Verification items for the finished model (mm, model axes). Round coordinates to 2 decimals unless told otherwise and drop trailing zeros. Write each question's results on one line, items separated by ' | '.
```python
from build123d import *

# Parameters (mm, degrees)
SKETCH2_R           = 12.7
SKETCH3_R           = 12.7
BOSS_EXTRUDE1_DEPTH = 50
SKETCH4_R           = 12.7
BOSS_EXTRUDE2_DEPTH = 35
SKETCH5_R           = 12.7
CUT_EXTRUDE1_DEPTH  = 634.359519319
SKETCH6_R           = 12.7
BOSS_EXTRUDE3_DEPTH = 40


with BuildPart() as part:
    # Sweep1: sweep along a curve in space
    with BuildLine() as sweep1_path:
        Line((-45.263841099, -132.462271612, 42.727197095), (-9.928000519, -34.667527384, 56.556883965))
        ThreePointArc((-45.263841099, -132.462271612, 42.727197095), (-49.367402807, -154.461340148, 40.074170619), (-46.268448436, -176.708192383, 38.254601427))
        Line((1.796645732, -332.656119714, 28.636985574), (-46.268448436, -176.708192383, 38.254601427))
        ThreePointArc((1.796645732, -332.656119714, 28.636985574), (9.693780672, -349.82422739, 28.096448926), (21.793712602, -364.33648604, 28.718411529))
        Line((159.088704017, -490.606286781, 40.497494579), (21.793712602, -364.33648604, 28.718411529))
        Line((159.088704017, -490.606286781, 40.497494579), (-47.055147145, -424.175155849, 20.376642682))
        ThreePointArc((-47.055147145, -424.175155849, 20.376642682), (-68.707848435, -412.682375082, 18.540437025), (-85.12514007, -394.403432402, 17.735499766))
        Line((-85.12514007, -394.403432402, 17.735499766), (-237.067860888, -150.281613827, 14.887673564))
        ThreePointArc((-237.067860888, -150.281613827, 14.887673564), (-245.860225068, -128.979461941, 14.519507014), (-247.259590984, -105.981912067, 13.905207225))
        Line((-247.259590984, -105.981912067, 13.905207225), (-240.877210012, -45.200693371, 12.011549601))
    # Sketch2 → Sweep1 (sweep)
    with BuildSketch(Plane(origin=(-240.877210012, -45.200693371, 12.011549601), x_dir=(0.994511346580908, -0.1045532802574024, -0.003974054509718908), z_dir=(0.10438154847039847, 0.9940550014184, -0.030970090312857718))):
        Circle(SKETCH2_R)
    sweep(path=sweep1_path.line, transition=Transition.RIGHT)

    # Sketch3 → Boss-Extrude1 (add)
    with BuildSketch(Plane(origin=(-240.877210012, -45.200693371, -19.129994659), x_dir=(-1, 0, 0), z_dir=(0, 0, -1))):
        with Locations((-1.013733677, 0)):
            Circle(SKETCH3_R)
    extrude(amount=-BOSS_EXTRUDE1_DEPTH)

    # Sketch4 → Boss-Extrude2 (add)
    with BuildSketch(Plane(origin=(-10.775481352, -33.333297989, 38.894650056), x_dir=(-0.9988573259328992, -0.0035999902794153107, 0.04765587581994679), z_dir=(-0.04779165649125455, 0.07524067855943051, -0.9960194766467865))):
        with Locations(Location((0, 0, 0), (0, 0, 90))):
            Circle(SKETCH4_R)
    extrude(amount=-BOSS_EXTRUDE2_DEPTH)

    # Sketch5 → Cut-Extrude1 (cut, through all)
    with BuildSketch(Plane(origin=(159.570708741, -491.36512975, 17.765263523), x_dir=(-0.9997755298808294, -0.0007068673202907124, -0.021175225857081564), z_dir=(0.02118702082660303, -0.03335573488518622, -0.9992189475278991))):
        Circle(SKETCH5_R)
    extrude(amount=-CUT_EXTRUDE1_DEPTH, mode=Mode.SUBTRACT)


with BuildPart() as body_2:
    # of the pieces the cut leaves, the one that is kept (cut_extrude1_keep)
    add(part.part.solids().sort_by_distance((-228.753597169, -51.353788927, 12.11141185))[0])

    # Sketch6 → Boss-Extrude3 (add)
    with BuildSketch(Plane(origin=(159.570708741, -491.36512975, 17.765263523), x_dir=(-0.9997755298808294, -0.0007068673202907124, -0.021175225857081564), z_dir=(0.02118702082660303, -0.03335573488518622, -0.9992189475278991))):
        with Locations(Location((0, 0, 0), (0, 0, 90))):
            Circle(SKETCH6_R)
    extrude(amount=-BOSS_EXTRUDE3_DEPTH)


solid = body_2.part
```
(1) Go/stop test with flat-tipped pins: pin 1 Ø6 at (x, y) = (-27.5, -300) entering from +Z; pin 2 Ø12 at (y, z) = (-300.5, 32.5) entering from -X; pin 3 Ø1.5 at (x, z) = (-110.5, 19) entering from -Y; pin 4 Ø7.5 at (x, y) = (-241, -43) entering from +Z. Record where each tip stops, or that it passes through.
Answer:
pin 1: through | pin 2: x = -153.61 | pin 3: y = -378.71 | pin 4: z = 30.87
(2) Thickness scan on L1, parallel to Y at x = -66.5, z = 14; L2, parallel to X at y = -193.5, z = 48.5; L3, parallel to X at y = -90, z = 45.5. Record the ranges inside material, lowest first.
Answer:
L1: -428.16 to -398.65 | L2: -47.45 to -35.16 | L3: -43.14 to -17.03
(3) Mould release check, pull along Y, two halves, no side actions. Record for faces 1 (the flat face through (-8.925, -36.143, 73.733)), 2 (the flat face through (-10.598, -33.51, 38.873)), 3 (the flat face through (-240, -45, 30.87)), 4 (the cylindrical face through (-257.436, -81.427, 13.791)): released by +Y, released by -Y, zero draft, split by the parting line, or undercut.
Answer:
face 1: released by -Y | face 2: released by +Y | face 3: zero draft | face 4: undercut
